The drawing under review shows one solid part. Ordinate dimensions are in mm from its lowest x, y, z. Give positions to 0.01 mm unless a question says otherwise; leave off trailing zeros. Write each loop counter-clockwise with the first axis right and the second up, starting at its lowest first coordinate (ties: lowest second). Pieces come first, ordered by that corner, then holes.
Q1. For line 1 (Y direction, x = 30.5, z = 53); line 2 (Z direction, x = 24, y = 76), list the stretches that pass through material, from the lowest coordinate up.
Q2. We need section C-C (x = 25). Write out the cut boundary in (y, z).
Q3. Insertion check: P1, Ø23, axis at y = 508, z = 51.89, coming from the +X side. The pin has a flat end and moves straight along its axis. Give the tip position at first contact, or say it passes through.
Q4. We need section A-A (y = 508). Write out the cut boundary in (x, z) (1 decimal).
Q5. We need section B-B (z = 44.5). Write out the cut boundary in (x, y) (1 decimal).
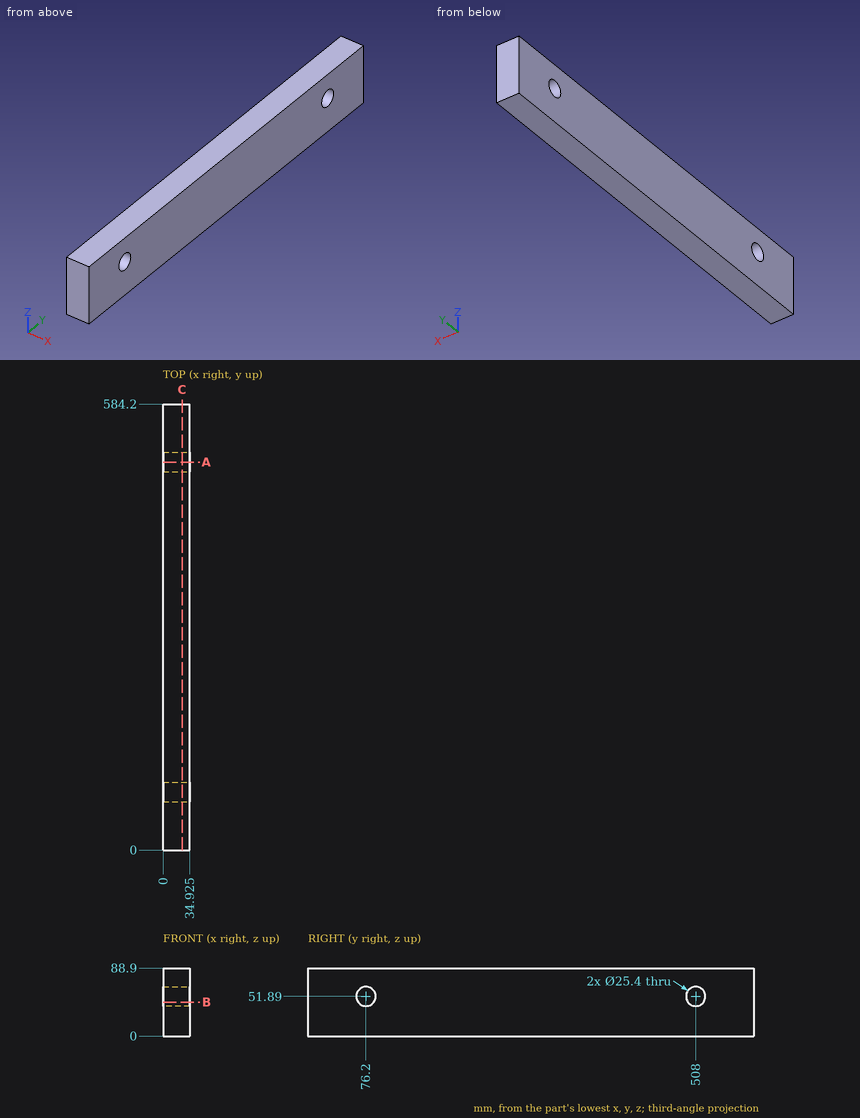
Computed:
1. line 1: y = 0 to 63.55, 88.85 to 495.35, 520.65 to 584.2
1. line 2: z = 0 to 39.19, 64.59 to 88.9
2. outline: (0, 0) - (584.2, 0) - (584.2, 88.9) - (0, 88.9) - close; hole circle Ø25.4 at (76.2, 51.89); hole circle Ø25.4 at (508, 51.89)
3. P1: passes through
4. outline: (0, 0) - (34.9, 0) - (34.9, 39.2) - (0, 39.2) - close; (0, 64.6) - (34.9, 64.6) - (34.9, 88.9) - (0, 88.9) - close
5. outline: (0, 0) - (34.9, 0) - (34.9, 65.9) - (0, 65.9) - close; (0, 86.5) - (34.9, 86.5) - (34.9, 497.7) - (0, 497.7) - close; (0, 518.3) - (34.9, 518.3) - (34.9, 584.2) - (0, 584.2) - close
